from build123d import *

# Parameters (mm, degrees)
SKETCH1_W           = 18
SKETCH1_H           = 4
BOSS_EXTRUDE1_DEPTH = 160
CUT_EXTRUDE1_DEPTH  = 160
SKETCH4_R           = 0.6
CUT_EXTRUDE2_DEPTH  = 160


with BuildPart() as part:
    # Sketch1 → Boss-Extrude1 (new body)
    with BuildSketch(Plane(origin=(0, 0, 0), x_dir=(1, 0, 0), z_dir=(0, 1, 0))):
        with Locations((-10.71526709, 13.305460186)):
            Rectangle(SKETCH1_W, SKETCH1_H)
    extrude(amount=BOSS_EXTRUDE1_DEPTH)

    # Sketch2 → Cut-Extrude1 (cut)
    with BuildSketch(Plane.XY):
        Polygon((-19.71526709, 18), (-19.71526709, 160), (-15.387039625, 160), (-17.100597756, 32.770358976), align=None)
        Polygon((-4.329936424, 32.770358976), (-6.043494554, 160), (-1.71526709, 160), (-1.71526709, 18), align=None)
    extrude(amount=-CUT_EXTRUDE1_DEPTH, mode=Mode.SUBTRACT)

    # Sketch4 → Cut-Extrude2 (cut)
    with BuildSketch(Plane.XY):
        with Locations((-10.71526709, 156.318807469)):
            Circle(SKETCH4_R)
    extrude(amount=-CUT_EXTRUDE2_DEPTH, mode=Mode.SUBTRACT)


solid = part.part
Could you check a few things on this model? Use its own coordinates, in mm. Round coordinates to 2 decimals unless told otherwise and drop trailing zeros. Order: outer loops, then holes, each group sorted by start corner. A loop starts at its lowest first (then second) coordinate and runs counter-clockwise, first axis right, second up.
(1) Imagine slicing it at B-B (y = 20.5). Write out the boundary of the cut face in (x, z).
Response values:
outline: (-19.27, -15.31) - (-2.16, -15.31) - (-2.16, -11.31) - (-19.27, -11.31) - close
(2) Imagine slicing it at A-A (z = -12.15). Write out the boundary of the cut face in (x, y), plus the area to 3 significant figures.
Response values:
outline: (-19.72, 0) - (-1.72, 0) - (-1.72, 18) - (-4.33, 32.77) - (-6.04, 160) - (-15.39, 160) - (-17.1, 32.77) - (-19.72, 18) - close; hole circle Ø1.2 at (-10.72, 156.32)
area: 1,960 mm2
(3) Please list where these lines run through material, in increasing order: line 1 along Y through (x, z) = (-11, -14.15); line 2 along X through (y, z) = (150, -12.4); line 3 along X through (y, z) = (144.5, -14.55).
Response values:
line 1: y = 0 to 155.79, 156.85 to 160
line 2: x = -15.52 to -5.91
line 3: x = -15.6 to -5.83
(4) Imagine slicing it at C-C (y = 68). Write out the boundary of the cut face in (x, z), plus the area to 3 significant figures.
Response values:
outline: (-16.63, -15.31) - (-4.8, -15.31) - (-4.8, -11.31) - (-16.63, -11.31) - close
area: 47.3 mm2
(5) I'm going to push a flat-ended pin straight in: pin 1 (2 mm diameter, centred on y = 34, z = -13, fed in from +X). Where does the tip first touch, or does it pass through?
Response values:
pin 1: stops at x = -4.33
